from build123d import *

# Parameters (mm, degrees)
SKETCH_1_R      = 2.5
EXTRUDE_1_DEPTH = 25
SKETCH_2_R      = 2
EXTRUDE_2_DEPTH = 8
SKETCH_3_R      = 4
EXTRUDE_3_DEPTH = 3


with BuildPart() as part:
    # 草图1 → 凸台-拉伸1 (new body)
    with BuildSketch(Plane(origin=(0, 0, 0), x_dir=(1, 0, 0), z_dir=(0, 1, 0))):
        Circle(SKETCH_1_R)
    extrude(amount=EXTRUDE_1_DEPTH)

    # 草图2 → 凸台-拉伸2 (add)
    with BuildSketch(Plane(origin=(0, 25, 0), x_dir=(1, 0, 0), z_dir=(0, 1, 0))):
        Circle(SKETCH_2_R)
    extrude(amount=EXTRUDE_2_DEPTH)

    # 草图3 → 凸台-拉伸3 (add)
    with BuildSketch(Plane.XZ):
        Circle(SKETCH_3_R)
    extrude(amount=EXTRUDE_3_DEPTH)


solid = part.part
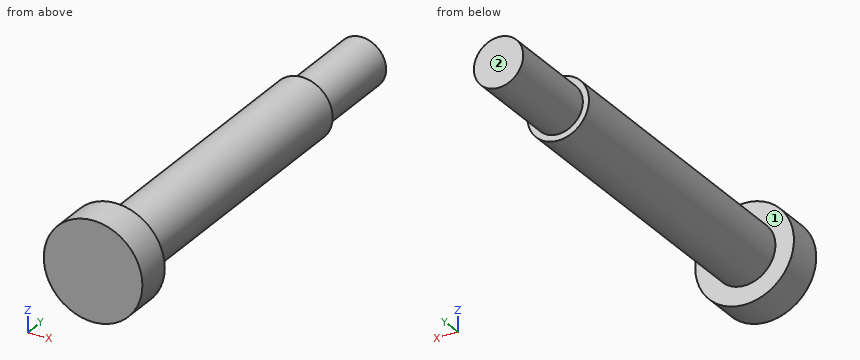
Can you work these out from the model? Positions are in its coordinate system, mm. Face numbers are marked on the shaded views. A direction names the side the tool comes from. Give positions to 0.01 mm unless a question says otherwise; leave off trailing zeros. Loops run counter-clockwise (first coordinate to the right, second up) from the corner with the lowest first, then second, coordinate; pieces in that order, holes last. Notation, with made-up numbers: M -40,19 L -9,19 A37 ccw -9,55 Z; hole C 9,54 d6. An arc over 180 degrees is marked long. One line per item, written item: value.
1) I'm going to push flat-ended pins straight in: pin 1 (4 mm diameter, centred on x = -1.5, z = -2, fed in from +Y); pin 2 (2 mm diameter, centred on y = 21, z = 0, fed in from -X); pin 3 (2 mm diameter, centred on x = -2.5, y = 16.5, fed in from -Z); pin 4 (4 mm diameter, centred on x = 3, y = 6.5, fed in from +Z). Where does each tip first touch, or does it pass through?
Geometry check:
pin 1: stops at y = 33
pin 2: stops at x = -2.5
pin 3: stops at z = -2
pin 4: stops at z = 2.29
2) Please list where these lines run through material, in increasing order: line 1 (Y direction, x = 2.5, z = -2); line 2 (X direction, y = 9, z = -1.5); line 3 (X direction, y = 5, z = 0).
Geometry check:
line 1: y = -3 to 0
line 2: x = -2 to 2
line 3: x = -2.5 to 2.5
3) Imagine slicing it at B-B on x = 0. Write out the boundary of the cut face in (y, z).
Geometry check:
outline: M -3,-4 L 0,-4 L 0,-2.5 L 25,-2.5 L 25,-2 L 33,-2 L 33,2 L 25,2 L 25,2.5 L 0,2.5 L 0,4 L -3,4 Z
4) On a 3-axis mill with a long thin cutter (end or side, diameter ignored), from which of +Z, -Z, +X, -X, +Y, -Y can I reach the whole of each face in a straight line? I mean the marked faces 1 and 2. Say none if no direction works.
Geometry check:
face 1: +Y
face 2: +Z, -Z, +X, -X, +Y
5) Imagine slicing it at C-C on y = 3. Write out the boundary of the cut face in (x, z), and give its area (3 significant figures).
Geometry check:
outline: C 0,0 d5
area: 19.6 mm²
6) Imagine slicing it at A-A on z = 0. Write out the boundary of the cut face in (x, y), and give its area (3 significant figures).
Geometry check:
outline: M -4,-3 L 4,-3 L 4,0 L 2.5,0 L 2.5,25 L 2,25 L 2,33 L -2,33 L -2,25 L -2.5,25 L -2.5,0 L -4,0 Z
area: 181 mm²
7) Imagine slicing it at D-D on y = 27.5. Write out the boundary of the cut face in (x, z).
Geometry check:
outline: C 0,0 d4
